from build123d import *

# Parameters (mm, degrees)
F1_DEPTH = 25


with BuildPart() as f1:
    # F0 (on Right) → F1 (new body, symmetric)
    with BuildSketch(Plane.YZ):
        with BuildLine():
            Line((0.5, 0), (10, 0))
            Line((10, 0), (10, 19))
            ThreePointArc((10, 19), (9.414214, 20.414214), (8, 21))
            Line((8, 21), (-3, 21))
            ThreePointArc((-3, 21), (-4.414214, 20.414214), (-5, 19))
            Line((-5, 19), (-5, 18))
            ThreePointArc((-5, 18), (-4.414214, 16.585786), (-3, 16))
            Line((-3, 16), (-2, 16))
            ThreePointArc((-2, 16), (-0.585786, 15.414214), (0, 14))
            Line((0, 14), (0, 13))
            ThreePointArc((0, 13), (-0.585786, 11.585786), (-2, 11))
            Line((-2, 11), (-8, 11))
            ThreePointArc((-8, 11), (-9.414214, 10.414214), (-10, 9))
            Line((-10, 9), (-10, 0))
            Line((-10, 0), (-0.5, 0))
            Line((-0.5, 0), (-0.5, 5))
            Line((-0.5, 5), (-6, 5))
            Line((-6, 5), (-6, 6))
            Line((-6, 6), (6, 6))
            Line((6, 6), (6, 5))
            Line((6, 5), (0.5, 5))
            Line((0.5, 5), (0.5, 0))
        make_face()
    extrude(amount=F1_DEPTH, both=True)


solid = f1.part
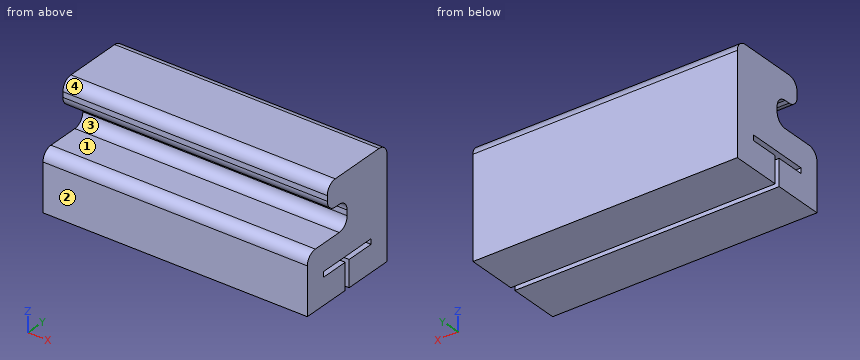
The listing builds one solid part. Answer for the finished solid, in the listing's coordinates (mm). Face numbers are marked on the shaded views. Give positions to 0.01 mm unless a question says otherwise; leave off trailing zeros. Order: outer loops, then holes, each group sorted by start corner. A loop starts at its lowest first (then second) coordinate and runs counter-clockwise, first axis right, second up. Notation, with made-up numbers: (-28.5, 82.5) - (4.5, 82.5) arc R24 cw to (4.5, 116.5) - close; hole circle Ø3 at (-39, -29). An arc over 180 degrees is marked (long way). One line per item, written item: value. Start each with the question number.
1) The mould has two halves that part along Z. Classify the marked faces 1, 2, 3 and 4: released by +Z, released by -Z, zero draft, split by the parting line, or undercut.
2) A cutting plane is placed at C-C on x = -10. Give the vertices of the cut face in (y, z), then the cut area to 3 significant figures.
3) Given pin 1 Ø1.6 at (x, y) = (10.5, -4) entering from +Z; pin 2 Ø1 at (x, z) = (-13.5, 18) entering from -Y; pin 3 Ø1.1 at (x, z) = (10.5, 13.5) entering from -Y, each flat-ended and moving along its own axis, determine where each tip first touches the part or whether it passes through.
4) A cutting plane is placed at D-D on z = 11.5. Give the vertices of the cut face in (x, y), then the cut area to 3 significant figures.
5) A cutting plane is placed at A-A on z = 2. Give the vertices of the cut face in (x, y).
6) A cutting plane is placed at B-B on y = 3.5. Give the vertices of the cut face in (x, z), then the cut area to 3 significant figures.
7) Find the intervals of material crossed by L1, parallel to Z at x = 20.5, y = -2.5; L2, parallel to Z at x = 16.5, y = 2.25; L3, parallel to Y at x = -3, z = 1.75, in increasing order.
Answer sheet:
1. face 1: undercut
1. face 2: zero draft
1. face 3: undercut
1. face 4: released by +Z
2. outline: (-10, 0) - (-0.5, 0) - (-0.5, 5) - (-6, 5) - (-6, 6) - (6, 6) - (6, 5) - (0.5, 5) - (0.5, 0) - (10, 0) - (10, 19) arc R2 ccw to (8, 21) - (-3, 21) arc R2 ccw to (-5, 19) - (-5, 18) arc R2 ccw to (-3, 16) - (-2, 16) arc R2 cw to (0, 14) - (0, 13) arc R2 cw to (-2, 11) - (-8, 11) arc R2 ccw to (-10, 9) - close
2. area: 326 mm2
3. pin 1: stops at z = 20.99
3. pin 2: stops at y = -5
3. pin 3: stops at y = 0
4. outline: (-25, -0.68) - (25, -0.68) - (25, 10) - (-25, 10) - close
4. area: 534 mm2
5. outline: (-25, -10) - (25, -10) - (25, -0.5) - (-25, -0.5) - close; (-25, 0.5) - (25, 0.5) - (25, 10) - (-25, 10) - close
6. outline: (-25, 0) - (25, 0) - (25, 5) - (-25, 5) - close; (-25, 6) - (25, 6) - (25, 21) - (-25, 21) - close
6. area: 1,000 mm2
7. L1: z = 0 to 5, 6 to 11, 16 to 21
7. L2: z = 0 to 5, 6 to 21
7. L3: y = -10 to -0.5, 0.5 to 10
